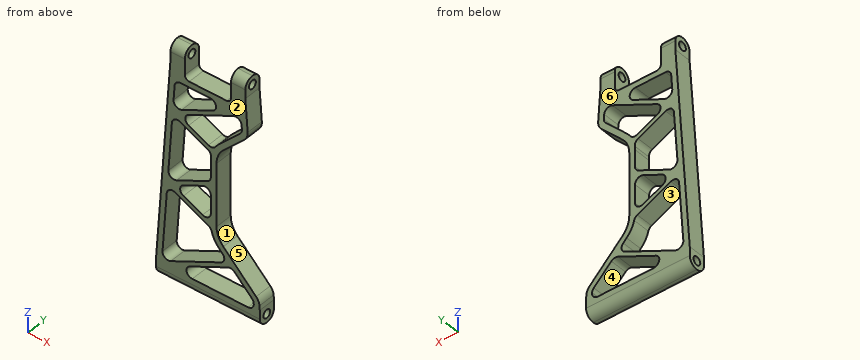
```python
from build123d import *

# Parameters (mm, degrees)
BOSS_EXTRUDE1_DEPTH     = 9.525
CUT_EXTRUDE2_DEPTH      = 139.148989433
CUT_EXTRUDE2_DEPTH_BACK = 139.148989433
SKETCH6_R               = 2.286
FILLET5_R               = 4.7625
FILLET6_R               = 12.7
FILLET7_R               = 6.35
CUT_EXTRUDE3_DEPTH      = 129.978879691
CUT_EXTRUDE3_DEPTH_BACK = 129.978879691
FILLET8_R               = 3.175
FILLET9_R               = 2.38125


# Some blends are built 0.0001 mm under size
with BuildPart() as part:
    # Sketch1 → Boss-Extrude1 (new body)
    with BuildSketch(Plane(origin=(0, 0, 0), x_dir=(1, 0, 0), z_dir=(0, 1, 0))):
        Polygon((-28.575, 4.7625), (-28.575, -4.7625), (-20.6375, -115.8875), (-20.6375, -125.4125), (-12.7, -125.4125), (-12.7, -109.5375), (12.7, -109.5375), (12.7, -125.4125), (20.6375, -125.4125), (20.6375, -115.8875), (22.111607143, -95.25), (4.7625, -77.900892857), (4.7625, -32.997321429), (28.234821429, -9.525), (28.575, -4.7625), (28.575, 4.7625), align=None)
    extrude(amount=BOSS_EXTRUDE1_DEPTH)

    # Sketch6 → Cut-Extrude2 (cut, two sides: drawn at the far end of the back side and taken through both)
    with BuildSketch(Plane.ZY.offset(28.575).offset(-CUT_EXTRUDE2_DEPTH_BACK)):
        with Locations((0, 4.7625)):
            Circle(SKETCH6_R)
        with Locations((120.65, 4.7625)):
            Circle(SKETCH6_R)
    extrude(amount=CUT_EXTRUDE2_DEPTH + CUT_EXTRUDE2_DEPTH_BACK, mode=Mode.SUBTRACT)

    # Fillet5
    fillet5_edges = [part.edges().sort_by_distance(p)[0] for p in [
        (0, 0, -4.7625),
        (0, 9.525, -4.7625),
        (16.66875, 0, 125.4125),
        (16.66875, 9.525, 125.4125),
        (-16.66875, 0, 125.4125),
        (-16.66875, 9.525, 125.4125),
    ]]
    fillet(fillet5_edges, radius=FILLET5_R - 0.0001)  # a hair under: the kernel refuses the full size

    # Fillet6
    fillet6_edges = [part.edges().sort_by_distance(p)[0] for p in [
        (4.7625, 4.7625, 32.997321429),
        (4.7625, 4.7625, 77.900892857),
    ]]
    fillet(fillet6_edges, radius=FILLET6_R)

    # Fillet7
    fillet7_edges = [part.edges().sort_by_distance(p)[0] for p in [
        (28.234821429, 4.7625, 9.525),
        (22.111607143, 4.7625, 95.25),
    ]]
    fillet(fillet7_edges, radius=FILLET7_R)

    # Sketch7 → Cut-Extrude3 (cut, two sides: drawn at the far end of the back side and taken through both)
    with BuildSketch(Plane.XZ.offset(-CUT_EXTRUDE3_DEPTH_BACK)):
        with BuildLine():
            ThreePointArc((-15.178464487, 106.3625), (-17.342073764, 105.511165186), (-18.345395859, 103.413709384))
            Line((-18.345395859, 103.413709384), (-18.929176024, 95.240787072))
            ThreePointArc((-18.929176024, 95.240787072), (-17.550554149, 92.391111633), (-14.394156229, 92.149449581))
            Line((-14.394156229, 92.149449581), (2.722039645, 100.322371894))
            ThreePointArc((2.722039645, 100.322371894), (4.450514376, 103.888871251), (1.353951221, 106.3625))
            Line((1.353951221, 106.3625), (-15.178464487, 106.3625))
        make_face()
        with BuildLine():
            Line((-10.652026542, 85.567257834), (2.949065003, 79.072785266))
            ThreePointArc((2.949065003, 79.072785266), (4.371896924, 81.621011779), (6.237179849, 83.865700766))
            Line((6.237179849, 83.865700766), (17.816220953, 95.444741871))
            ThreePointArc((17.816220953, 95.444741871), (18.545921053, 96.580119743), (18.738088295, 97.916015285))
            Line((18.738088295, 97.916015285), (18.355750526, 103.268744039))
            ThreePointArc((18.355750526, 103.268744039), (16.767104452, 103.883635913), (15.089301508, 103.588906124))
            Line((15.089301508, 103.588906124), (-10.652026542, 91.297514046))
            ThreePointArc((-10.652026542, 91.297514046), (-12.458938118, 88.43238594), (-10.652026542, 85.567257834))
        make_face()
        with BuildLine():
            ThreePointArc((-15.303455952, 85.149509664), (-18.268395024, 85.028592375), (-19.838475748, 82.510590942))
            Line((-19.838475748, 82.510590942), (-21.768351953, 55.492324069))
            ThreePointArc((-21.768351953, 55.492324069), (-20.389730078, 52.642648631), (-17.233332157, 52.400986579))
            Line((-17.233332157, 52.400986579), (1.5875, 61.38786662))
            Line((1.5875, 61.38786662), (1.5875, 72.640380615))
            ThreePointArc((1.5875, 72.640380615), (1.727944926, 74.747369375), (2.146794694, 76.817077393))
            Line((2.146794694, 76.817077393), (-15.303455952, 85.149509664))
        make_face()
        with BuildLine():
            Line((1.5875, 38.618768332), (1.5875, 58.749077544))
            Line((1.5875, 58.749077544), (-13.49120247, 51.549051044))
            ThreePointArc((-13.49120247, 51.549051044), (-15.298114047, 48.683922938), (-13.49120247, 45.818794832))
            Line((-13.49120247, 45.818794832), (1.5875, 38.618768332))
        make_face()
        with BuildLine():
            ThreePointArc((-18.142631881, 45.401046662), (-21.107570953, 45.280129373), (-22.677651676, 42.76212794))
            Line((-22.677651676, 42.76212794), (-25.022707709, 9.93134348))
            ThreePointArc((-25.022707709, 9.93134348), (-23.644085834, 7.081668041), (-20.487687914, 6.84000599))
            Line((-20.487687914, 6.84000599), (11.26695768, 22.002735688))
            Line((11.26695768, 22.002735688), (6.237179849, 27.032513519))
            ThreePointArc((6.237179849, 27.032513519), (3.290050222, 31.105401057), (1.764238406, 35.895587299))
            Line((1.764238406, 35.895587299), (-18.142631881, 45.401046662))
        make_face()
        with BuildLine():
            ThreePointArc((-9.987271687, 9.215128106), (-11.715746418, 5.648628749), (-8.619183264, 3.175))
            Line((-8.619183264, 3.175), (22.095428773, 3.175))
            ThreePointArc((22.095428773, 3.175), (24.419093959, 4.186390723), (25.262360145, 6.576209384))
            Line((25.262360145, 6.576209384), (25.236657334, 6.936048729))
            ThreePointArc((25.236657334, 6.936048729), (24.957868459, 8.028648627), (24.314789993, 8.954903375))
            Line((24.314789993, 8.954903375), (13.052944458, 20.21674891))
            Line((13.052944458, 20.21674891), (-9.987271687, 9.215128106))
        make_face()
    extrude(amount=CUT_EXTRUDE3_DEPTH + CUT_EXTRUDE3_DEPTH_BACK, mode=Mode.SUBTRACT)

    # Fillet8
    # the kernel refuses this fillet: 3.175 mm, written as the material it adds along each edge
    with BuildSketch(Plane(origin=(2.146794694, 0, 76.817077393), x_dir=(-0.19425863373245403, 0, -0.9809503469699169), z_dir=(0, 1, 0))) as fillet8_piece_1:
        with BuildLine():
            CenterArc((2.468233166, 3.167061169), FILLET8_R, 194.322890181, 71.624501931)
            Line((-0.608078232, 2.381610227), (0, 0))
            ThreePointArc((0, 0), (1.121924166, 0.039694156), (2.243848333, 0))
        make_face()
    extrude(amount=9.525)
    with BuildSketch(Plane(origin=(1.5875, 0, 61.38786662), x_dir=(0, 0, 1), z_dir=(0, 1, 0))) as fillet8_piece_2:
        with BuildLine():
            CenterArc((FILLET8_R * 0.630656469631, -FILLET8_R), FILLET8_R, 90, 64.475691518)
            Line((-FILLET8_R * 0.271746083545, -FILLET8_R * 0.569106008372), (0, 0))
            Line((0, 0), (FILLET8_R * 0.630656469631, 0))
        make_face()
    extrude(amount=9.525)
    with BuildSketch(Plane(origin=(2.949065003, 9.525, 79.072785266), x_dir=(0.482167275870273, 0, 0.8760791734083397), z_dir=(0, -1, 0))) as fillet8_piece_3:
        with BuildLine():
            CenterArc((2.997736865, 3.163282633), FILLET8_R, 183.302737657, 81.773303175)
            Line((-0.171989666, 2.980365394), (0, 0))
            ThreePointArc((0, 0), (1.362607666, 0.058586837), (2.725215332, 0))
        make_face()
    extrude(amount=9.525)
    with BuildSketch(Plane(origin=(18.355750526, 0, 103.268744039), x_dir=(-0.9990488574203268, 0, -0.04360482183359276), z_dir=(0, 1, 0))) as fillet8_piece_4:
        with BuildLine():
            CenterArc((3.095288472, -2.922058213), FILLET8_R, 66.97485618, 111.438691702)
            Line((-0.078494517, -2.834157465), (-0.395872815, -2.82536739))
            Line((-0.395872815, -2.82536739), (-0.317378299, 0.008790075))
            Line((-0.317378299, 0.008790075), (-0.200752777, 0.245976772))
            ThreePointArc((-0.200752777, 0.245976772), (3.373566927, 0.754496314), (4.461327625, 0.292205821))
            Line((4.461327625, 0.292205821), (4.337142248, 0))
        make_face()
    extrude(amount=9.525)
    with BuildSketch(Plane(origin=(1.764238406, 9.525, 35.895587299), x_dir=(-0.9024025531760991, 0, 0.4308939916281702), z_dir=(0, -1, 0))) as fillet8_piece_5:
        with BuildLine():
            CenterArc((1.589224556, 3.175), FILLET8_R, 219.319739753, 50.680260247)
            ThreePointArc((-0.867025133, 1.163169374), (-0.420218411, 0.591494135), (0, 0))
            Line((0, 0), (1.589224556, 0))
        make_face()
    extrude(amount=9.525)
    with BuildSketch(Plane(origin=(11.26695768, 9.525, 22.002735688), x_dir=(-0.7071067811865471, 0, 0.7071067811865479), z_dir=(0, -1, 0))) as fillet8_piece_6:
        with BuildLine():
            CenterArc((FILLET8_R * 1.4143306163, FILLET8_R), FILLET8_R, 160.524308482, 109.475691518)
            Line((FILLET8_R * 0.471547588134, FILLET8_R * 1.33340690126), (0, 0))
            Line((0, 0), (FILLET8_R * 1.4143306163, 0))
        make_face()
    extrude(amount=9.525)
    with BuildSketch(Plane(origin=(1.5875, 0, 58.749077544), x_dir=(-0.9024025531760999, 0, -0.4308939916281688), z_dir=(0, 1, 0))) as fillet8_piece_7:
        with BuildLine():
            CenterArc((FILLET8_R * 1.58564931647, -FILLET8_R), FILLET8_R, 90, 115.524308482)
            Line((FILLET8_R * 0.683246763298, -FILLET8_R * 1.43089399163), (0, 0))
            Line((0, 0), (FILLET8_R * 1.58564931647, 0))
        make_face()
    extrude(amount=9.525)
    with BuildSketch(Plane(origin=(1.5875, 9.525, 38.618768332), x_dir=(0, 0, 1), z_dir=(0, -1, 0))) as fillet8_piece_8:
        with BuildLine():
            CenterArc((FILLET8_R * 1.58564931647, FILLET8_R), FILLET8_R, 154.475691518, 115.524308482)
            Line((FILLET8_R * 0.683246763298, FILLET8_R * 1.43089399163), (0, 0))
            Line((0, 0), (FILLET8_R * 1.58564931647, 0))
        make_face()
    extrude(amount=9.525)
    with BuildSketch(Plane(origin=(13.052944458, 9.525, 20.21674891), x_dir=(-0.9024025531761012, 0, -0.4308939916281661), z_dir=(0, -1, 0))) as fillet8_piece_9:
        with BuildLine():
            CenterArc((FILLET8_R * 0.707048259068, FILLET8_R), FILLET8_R, 199.475691518, 70.524308482)
            Line((-FILLET8_R * 0.235734769096, FILLET8_R * 0.666593098742), (0, 0))
            Line((0, 0), (FILLET8_R * 0.707048259068, 0))
        make_face()
    extrude(amount=9.525)

    # Fillet9
    fillet9_edges = [part.edges().sort_by_distance(p)[0] for p in [
        (12.7, 4.7625, 109.5375),
        (-12.7, 4.7625, 109.5375),
    ]]
    fillet(fillet9_edges, radius=FILLET9_R)


solid = part.part
```
Design review of the part built by this model. Coordinates are the model's own, in mm. Face numbers are marked on the shaded views. A direction names the side the tool comes from. Coordinates: 2 decimals unless noted, no trailing zeros. Order: outer loops, then holes, each group sorted by start corner. A loop starts at its lowest first (then second) coordinate and runs counter-clockwise, first axis right, second up.
1) For the marked faces 4, 5 and 6, list the 3-axis set-ups (+Z, -Z, +X, -X, +Y, -Y) from which the entire face can be reached by the end or side of a thin tool; tool diameter is ignored.
2) Wall thickness on line 1 along Y through (x, z) = (-10, 0) (1 decimal); line 2 along X through (y, z) = (8.5, 97.5); line 3 along Z through (x, y) = (11.5, 8.25) (3 decimals): over which ranges is each line inside the solid? List them lowest first.
3) Take a section at A-A, the plane z = 23.5. Give the boundary of the cut face in (x, y) (3 decimals), and give its area (3 significant figures).
4) Clearance check with flat-ended pins moving along their axes: pin 1 (3 mm diameter, centred on y = 2.5, z = 119, fed in from +X); pin 2 (3 mm diameter, centred on y = 5.5, z = 50.5, fed in from -X); pin 3 (4.5 mm diameter, centred on y = 4, z = 69.5, fed in from -X). State where each tip first meets the part, or that it passes through.
5) Mouldability with a two-part tool opening along X and no side actions: class the marked faces 1, 2 and 3 as +X half, -X half, draft (parallel to the pull), parting line (faces both ways), or undercut.
Returned:
1. face 4: +Y, -Y
1. face 5: +X, +Y, -Y
1. face 6: +Z, -Z, +X, -X, +Y
2. line 1: y = 0 to 2.5, 7 to 9.5
2. line 2: x = -21.95 to -18.77, -3.19 to 2.34, 18.74 to 21.92
2. line 3: z = -3.243 to 3.175, 19.43 to 26.26, 84.638 to 89.129, 101.875 to 109.851
3. outline: (-27.237, 0) - (-24.054, 0) - (-24.054, 9.525) - (-27.237, 9.525) - close; (8.971, 0) - (14.26, 0) - (14.26, 9.525) - (8.971, 9.525) - close
3. area: 80.7 mm2
4. pin 1: stops at x = 20.64
4. pin 2: stops at x = -25.42
4. pin 3: stops at x = -24.11
5. face 1: +X half
5. face 2: draft
5. face 3: undercut
